from build123d import *

# Parameters (mm, degrees)
ESQUISSE1_R             = 8
BOSS_EXTRU_1_DEPTH      = 5
ESQUISSE2_W             = 30
ESQUISSE2_H             = 12
BOSS_EXTRU_2_DEPTH      = 10.5
ESQUISSE4_W             = 30
ESQUISSE4_H             = 5
BOSS_EXTRU_3_DEPTH      = 45
ENL_V_START             = -10
ESQUISSE6_R             = 8
ENL_V_MAT_EXTRU_3_DEPTH = 10
ESQUISSE8_W             = 8
ESQUISSE8_H             = 8
ESQUISSE8_R             = 2.3
BOSS_EXTRU_4_DEPTH      = 8
ENL_V_MAT_EXTRU_4_DEPTH = 2
ENL_V_MAT_EXTRU_5_DEPTH = 50
ENL_V_MAT_EXTRU_6_DEPTH = 50
BOSS_EXTRU_5_DEPTH      = 10.5


with BuildPart() as part:
    # Esquisse1 → Boss.-Extru.1 (new body)
    with BuildSketch(Plane.XY):
        Polygon((0, 0), (15, 0), (15, 45), (-15, 45), (-15, 0), align=None)
        with Locations((0, 28)):
            Circle(ESQUISSE1_R, mode=Mode.SUBTRACT)
    extrude(amount=-BOSS_EXTRU_1_DEPTH)

    # Esquisse2 → Boss.-Extru.2 (add)
    with BuildSketch(Plane(origin=(0, 0, -5), x_dir=(-1, 0, 0), z_dir=(0, 0, -1))):
        with Locations((0, 6)):
            Rectangle(ESQUISSE2_W, ESQUISSE2_H)
    extrude(amount=BOSS_EXTRU_2_DEPTH)

    # Esquisse4 → Boss.-Extru.3 (add)
    with BuildSketch(Plane.XZ):
        with Locations((0, -18)):
            Rectangle(ESQUISSE4_W, ESQUISSE4_H)
    extrude(amount=-BOSS_EXTRU_3_DEPTH)

    # Esquisse6 → Enlèv. mat.-Extru.3 (cut)
    with BuildSketch(Plane(origin=(0, 0, -20.5), x_dir=(-1, 0, 0), z_dir=(0, 0, -1)).offset(ENL_V_START)):
        with Locations(Location((0, 28, 0), (0, 0, 180))):
            Circle(ESQUISSE6_R)
    extrude(amount=ENL_V_MAT_EXTRU_3_DEPTH, mode=Mode.SUBTRACT)

    # Esquisse8 → Boss.-Extru.4 (add)
    # profile 1 of 4: a face of its own
    with BuildSketch(Plane.XZ):
        with Locations((-11, 4)):
            Rectangle(ESQUISSE8_W, ESQUISSE8_H)
        with Locations(Location((-11, 4, 0), (0, 0, 270))):
            Circle(ESQUISSE8_R, mode=Mode.SUBTRACT)
    # profile 2 of 4: a face of its own
    with BuildSketch(Plane.XZ):
        with Locations((11, 4)):
            Rectangle(ESQUISSE8_W, ESQUISSE8_H)
        with Locations(Location((11, 4, 0), (0, 0, 270))):
            Circle(ESQUISSE8_R, mode=Mode.SUBTRACT)
    # profile 3 of 4: a face of its own
    with BuildSketch(Plane.XZ):
        with Locations((-11, -24.5)):
            Rectangle(ESQUISSE8_W, ESQUISSE8_H)
        with Locations(Location((-11, -24.5, 0), (0, 0, 270))):
            Circle(ESQUISSE8_R, mode=Mode.SUBTRACT)
    # profile 4 of 4: a face of its own
    with BuildSketch(Plane.XZ):
        with Locations((11, -24.5)):
            Rectangle(ESQUISSE8_W, ESQUISSE8_H)
        with Locations(Location((11, -24.5, 0), (0, 0, 270))):
            Circle(ESQUISSE8_R, mode=Mode.SUBTRACT)
    extrude(amount=-BOSS_EXTRU_4_DEPTH)

    # Esquisse9 → Enlèv. mat.-Extru.4 (cut)
    with BuildSketch(Plane.XZ):
        Polygon((-15, 8), (-15, -28.5), (-7, -28.5), (-7, -20.5), (7, -20.5), (7, -28.5), (15, -28.5), (15, 8), (7, 8), (7, 0), (-7, 0), (-7, 8), align=None)
    extrude(amount=-ENL_V_MAT_EXTRU_4_DEPTH, mode=Mode.SUBTRACT)

    # Esquisse10 → Enlèv. mat.-Extru.5 (cut)
    with BuildSketch(Plane.ZY.offset(15)):
        with BuildLine():
            Line((-13.25, 2), (-7.25, 2))
            Line((-7.25, 2), (-7.25, 5.5))
            ThreePointArc((-7.25, 5.5), (-10.25, 8.5), (-13.25, 5.5))
            Line((-13.25, 5.5), (-13.25, 2))
        make_face()
    extrude(amount=-ENL_V_MAT_EXTRU_5_DEPTH, mode=Mode.SUBTRACT)

    # Esquisse11 → Enlèv. mat.-Extru.6 (cut)
    with BuildSketch(Plane.XY):
        Polygon((-9, 45), (-15, 45), (-15, 39), align=None)
        Polygon((15, 45), (9, 45), (15, 39), align=None)
    extrude(amount=-ENL_V_MAT_EXTRU_6_DEPTH, mode=Mode.SUBTRACT)

    # Esquisse12 → Boss.-Extru.5 (add)
    with BuildSketch(Plane(origin=(0, 0, -5), x_dir=(-1, 0, 0), z_dir=(0, 0, -1))):
        Polygon((0, 12), (15, 12), (15, 20), align=None)
    extrude(amount=BOSS_EXTRU_5_DEPTH)


solid = part.part
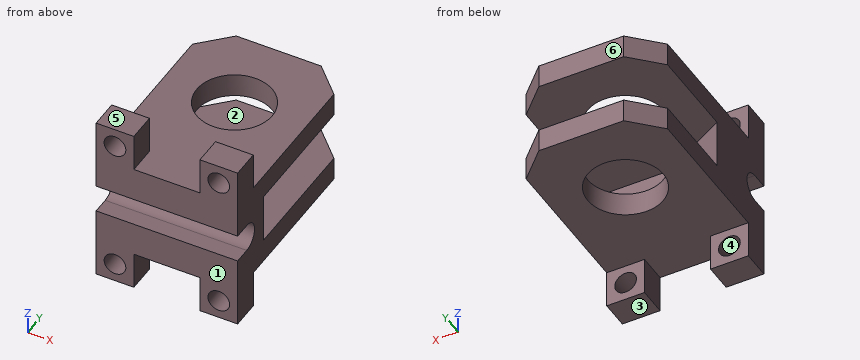
Here's how the part is built. I have some questions about the finished solid (model axes, mm). Face numbers are marked on the shaded views. A direction names the side the tool comes from. Coordinates: 2 decimals unless noted, no trailing zeros. Loops run counter-clockwise (first coordinate to the right, second up) from the corner with the lowest first, then second, coordinate; pieces in that order, holes last.
1. If we mould it in two halves opening along Z, with no side actions, what happens to the marked faces 3, 4, 5 and 6? For each: pulls with the +Z half, pulls with the -Z half, needs draft (parallel to the pull), parting line crosses it, or undercut.
2. Imagine slicing it at D-D, the plane z = -10.25. Please give me the cut outline in (x, y).
3. For the marked faces 1 and 2, which set-ups out of +Z, -Z, +X, -X, +Y, -Y let a thin tool reach every point of the face, with its end or its side?
4. For P1, Ø6, axis at x = 11, z = 3.5, coming from the +Y side; P2, Ø3, axis at x = 2, y = 12.5, coming from the -Z side; P3, Ø1.8, axis at x = -5, y = 3.5, coming from the +Z side, each with a flat end and sliding along its axis, tell me the tip position at first contact or that it passes through.
5. Imagine slicing it at B-B, the plane y = 37.5. Please give me the cut outline in (x, z).
6. Imagine slicing it at C-C, the plane x = 11. Please give me the cut outline in (y, z).
7. Imagine slicing it at A-A, the plane z = 4. Please give me the cut outline in (x, y), and give its area (3 significant figures).
8. I need wall thicknesses on L1, parallel to X at y = 3.8, z = 4; L2, parallel to X at y = 7.5, z = 6.5; L3, parallel to Z at x = 4, y = 15. Which ranges of each line are inside material? Lowest first, please.
Taken from the geometry:
1. face 3: pulls with the -Z half
1. face 4: undercut
1. face 5: pulls with the +Z half
1. face 6: needs draft
2. outline: (-15, 8.5) - (15, 8.5) - (15, 12) - (0, 12) - (-15, 20) - close
3. face 1: +Z, -Z, +X, -X, -Y
3. face 2: +X, +Y
4. P1: stops at y = 8
4. P2: stops at z = -20.5
4. P3: stops at z = 0
5. outline: (-15, -20.5) - (15, -20.5) - (15, -15.5) - (-15, -15.5) - close; (-15, -5) - (15, -5) - (15, 0) - (-15, 0) - close
6. outline: (2, -28.5) - (8, -28.5) - (8, -26.8) - (2, -26.8) - close; (2, -22.2) - (8, -22.2) - (8, -20.5) - (43, -20.5) - (43, -15.5) - (12, -15.5) - (12, -5) - (43, -5) - (43, 0) - (8, 0) - (8, 1.7) - (2, 1.7) - (2, -7.25) - (5.5, -7.25) arc R3 cw to (5.5, -13.25) - (2, -13.25) - close; (2, 6.3) - (8, 6.3) - (8, 8) - (2, 8) - close
7. outline: (-15, 2) - (-13.3, 2) - (-13.3, 8) - (-15, 8) - close; (-8.7, 2) - (-7, 2) - (-7, 8) - (-8.7, 8) - close; (7, 2) - (8.7, 2) - (8.7, 8) - (7, 8) - close; (13.3, 2) - (15, 2) - (15, 8) - (13.3, 8) - close
7. area: 40.8 mm2
8. L1: x = -15 to -13.3, -8.7 to -7, 7 to 8.7, 13.3 to 15
8. L2: x = -15 to -7, 7 to 15
8. L3: z = -20.5 to -15.5, -5 to 0
